from build123d import *

# Parameters (mm, degrees)
ODGI_CIE_BAZOWE1_DEPTH  = 15
OTW_R_POD_RUB_M61_D     = 6.6
OTW_R_POD_RUB_M61_DEPTH = 10
OTW_R_POD_RUB_M61_TIP   = 1.982840043
ZAOKR_GLENIE1_R         = 2


# Sheet-metal steps are written as plain solids
with BuildPart() as part:
    # Szkic1 → Odgięcie bazowe1 (new, symmetric)
    with BuildSketch(Plane.XY):
        with BuildLine():
            Line((15, 0), (3.5, 0))
            ThreePointArc((3.5, 0), (1.025126266, -1.025126266), (0, -3.5))
            Line((0, -3.5), (0, -25))
            Line((0, -25), (1.5, -25))
            Line((1.5, -25), (1.5, -3.5))
            ThreePointArc((1.5, -3.5), (2.085786438, -2.085786438), (3.5, -1.5))
            Line((3.5, -1.5), (15, -1.5))
            Line((15, -1.5), (15, 0))
        make_face()
    extrude(amount=ODGI_CIE_BAZOWE1_DEPTH, both=True)

    # Otwór pod śrubę M61
    with Locations(Plane.ZY):
        with Locations((-9, -15), (7, -15)):
            Hole(OTW_R_POD_RUB_M61_D / 2, depth=OTW_R_POD_RUB_M61_DEPTH)
            with Locations((0, 0, -(OTW_R_POD_RUB_M61_DEPTH + OTW_R_POD_RUB_M61_TIP / 2))):  # 118° drill point
                Cone(0, OTW_R_POD_RUB_M61_D / 2, OTW_R_POD_RUB_M61_TIP, mode=Mode.SUBTRACT)

    # Zaokrąglenie1
    zaokr_glenie1_edges = [part.edges().sort_by_distance(p)[0] for p in [
        (0.75, -25, 15),
        (0.75, -25, -15),
        (15, -0.75, 15),
        (15, -0.75, -15),
    ]]
    fillet(zaokr_glenie1_edges, radius=ZAOKR_GLENIE1_R)


solid = part.part
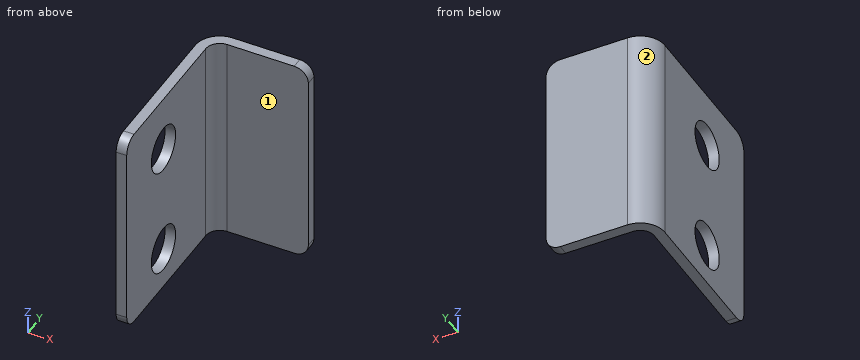
Here's how the part is built. I have some questions about the finished solid (model axes, mm). Face numbers are marked on the shaded views. A direction names the side the tool comes from. Round coordinates to 2 decimals unless told otherwise and drop trailing zeros. Order: outer loops, then holes, each group sorted by start corner. A loop starts at its lowest first (then second) coordinate and runs counter-clockwise, first axis right, second up. Notation, with made-up numbers: (60.25, 4.25) -> (109.25, 4.25) arc R34 ccw to (109.25, 35.25) -> close; hole circle Ø9 at (78, 78). An arc over 180 degrees is marked (long way). Return JSON: item names as keys, results as strings.
Q1. If we section it at D-D on x = 9.5: List the corners of the cut face in (y, z) for me.
Filled sheet:
{"outline": "(-1.5, -15) -> (0, -15) -> (0, 15) -> (-1.5, 15) -> close"}
Q2. If we section it at B-B on z = -9: List the corners of the cut face in (x, y) for me, plus the area to 3 significant figures.
Filled sheet:
{"outline": "(0, -25) -> (1.5, -25) -> (1.5, -18.3) -> (0, -18.3) -> close; (0, -11.7) -> (1.5, -11.7) -> (1.5, -3.5) arc R2 cw to (3.5, -1.5) -> (15, -1.5) -> (15, 0) -> (3.5, 0) arc R3.5 ccw to (0, -3.5) -> close", "area": "46.1 mm^2"}
Q3. For pin 1 Ø3 at (x, z) = (13.5, -6) entering from -Y; pin 2 Ø4 at (y, z) = (-15, -9) entering from -X; pin 3 Ø10 at (y, z) = (-16.5, 5) entering from +X, each with a flat end and sliding along its axis, tell me the tip position at first contact or that it passes through.
Filled sheet:
{"pin 1": "stops at y = -1.5", "pin 2": "passes through", "pin 3": "stops at x = 1.5"}
Q4. Which directions (+Z, -Z, +X, -X, +Y, -Y) give clear straight access to the entire face, cutting with the end or side of a thin tool? Please do the marked faces 1 and 2.
Filled sheet:
{"face 1": "+Z, -Z, +X, -Y", "face 2": "+Z, -Z, -X, +Y"}
Q5. I need wall thicknesses on line 1 along X through (y, z) = (-15.75, -12.5); line 2 along Y through (x, z) = (4.5, 13); line 3 along Y through (x, z) = (0.7, 7). Which ranges of each line are inside material? Lowest first, please. Write a range as from..to.
Filled sheet:
{"line 1": "x = 0..1.5", "line 2": "y = -1.5..0", "line 3": "y = -25..-18.3, -11.7..-1.4"}
Q6. If we section it at C-C on z = -5.25: List the corners of the cut face in (x, y) for me, plus the area to 3 significant figures.
Filled sheet:
{"outline": "(0, -25) -> (1.5, -25) -> (1.5, -3.5) arc R2 cw to (3.5, -1.5) -> (15, -1.5) -> (15, 0) -> (3.5, 0) arc R3.5 ccw to (0, -3.5) -> close", "area": "56.0 mm^2"}
Q7. If we section it at A-A on y = -15: List the corners of the cut face in (x, z) for me, plus the area to 3 significant figures.
Filled sheet:
{"outline": "(0, -15) -> (1.5, -15) -> (1.5, -12.3) -> (0, -12.3) -> close; (0, -5.7) -> (1.5, -5.7) -> (1.5, 3.7) -> (0, 3.7) -> close; (0, 10.3) -> (1.5, 10.3) -> (1.5, 15) -> (0, 15) -> close", "area": "25.2 mm^2"}
